Check sheet for the drawn part. Datum: minimum x, y, z corner. Units: mm. A direction names the side the tool comes from. Coordinates: 2 decimals unless noted, no trailing zeros. Order: outer loops, then holes, each group sorted by start corner. A loop starts at its lowest first (then second) coordinate and runs counter-clockwise, first axis right, second up. Notation, with made-up numbers: (34, 85.25) - (83, 85.25) arc R12 ccw to (83, 91.25) - close; hole circle Ø3 at (48, -13). An arc over 180 degrees is marked (long way). Put each result on its own line as item: value.
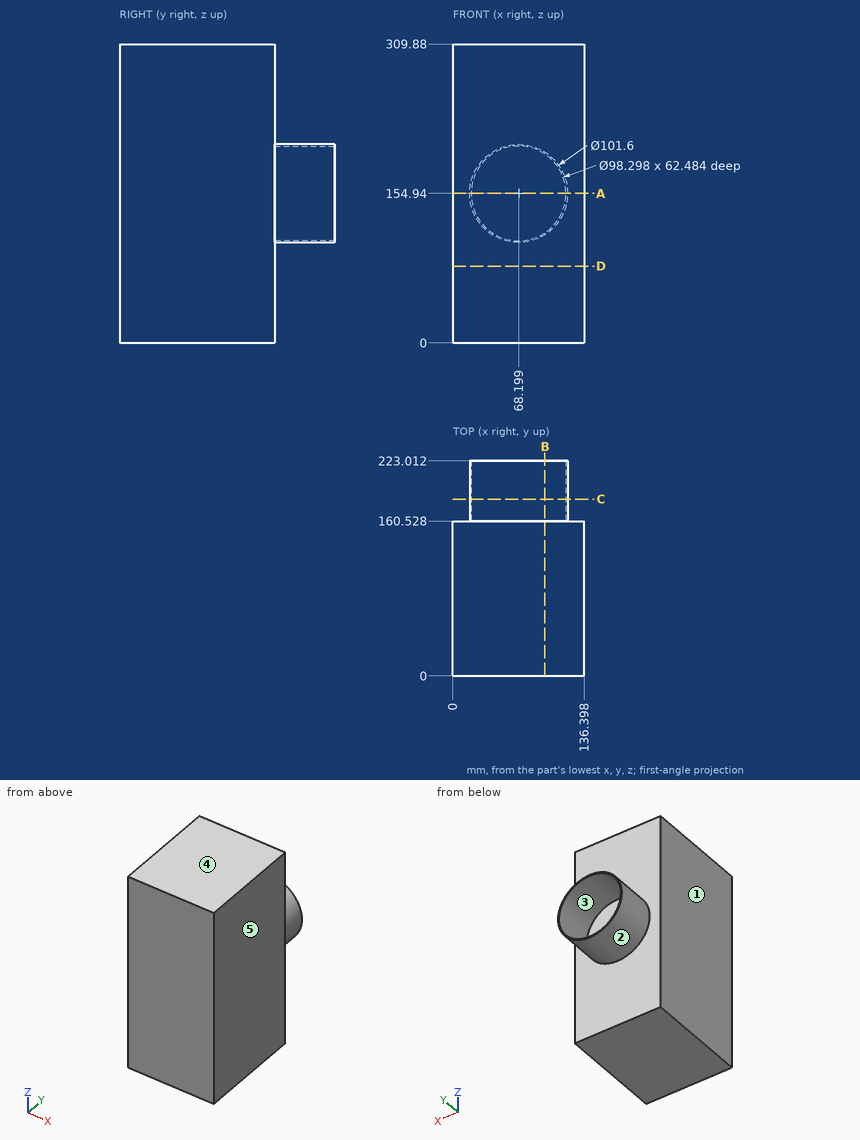
Q1. Thickness scan on L1, parallel to X at y = 192, z = 154.94; L2, parallel to Y at x = 128.5, z = 84.5; L3, parallel to Z at x = 75, y = 207.5. Record the ranges inside material, lowest first. Write a range as [from, to].
Answer block:
L1: x = [17.4, 19.05], [117.35, 119]
L2: y = [0, 160.53]
L3: z = [104.6, 106.26], [203.62, 205.28]
Q2. Section check C-C on y = 183.5. Record the boundary of the cut face in (x, z), then the cut area to 3 significant figures.
Answer block:
outline: circle Ø101.6 at (68.2, 154.94); hole circle Ø98.3 at (68.2, 154.94)
area: 518 mm^2
Q3. Access from +Z, -Z, +X, -X, +Y, -Y to the whole of each face (thin tool, end or side, straight path). Record for the marked faces 1 and 2.
Answer block:
face 1: +Z, -Z, -X, +Y, -Y
face 2: +Y
Q4. Depth check by flat-ended pin: pin 1 Ø4 at (x, z) = (41.5, 216) entering from +Y. Enter the tip coordinate at first touch or a pass-through.
Answer block:
pin 1: stops at y = 160.53
Q5. Draft check along Z on the marked faces 3, 4 and 5. Enter one of: pulls with the +Z half, pulls with the -Z half, needs draft (parallel to the pull), parting line crosses it, or undercut.
Answer block:
face 3: undercut
face 4: pulls with the +Z half
face 5: needs draft
Q6. Section check B-B on x = 95.5. Record the boundary of the cut face in (y, z).
Answer block:
outline: (0, 0) - (160.53, 0) - (160.53, 112.1) - (223.01, 112.1) - (223.01, 114.07) - (160.53, 114.07) - (160.53, 195.81) - (223.01, 195.81) - (223.01, 197.78) - (160.53, 197.78) - (160.53, 309.88) - (0, 309.88) - close
Q7. Section check D-D on z = 79.5. Record the boundary of the cut face in (x, y), then the cut area to 3 significant figures.
Answer block:
outline: (0, 0) - (136.4, 0) - (136.4, 160.53) - (0, 160.53) - close
area: 21,900 mm^2
Q8. Section check A-A on z = 154.94. Record the boundary of the cut face in (x, y).
Answer block:
outline: (0, 0) - (136.4, 0) - (136.4, 160.53) - (119, 160.53) - (119, 223.01) - (117.35, 223.01) - (117.35, 160.53) - (19.05, 160.53) - (19.05, 223.01) - (17.4, 223.01) - (17.4, 160.53) - (0, 160.53) - close
